Check sheet for the drawn part. Datum: minimum x, y, z corner. Units: mm. A direction names the side the tool comes from. Coordinates: 2 decimals unless noted, no trailing zeros. Order: outer loops, then holes, each group sorted by start corner. A loop starts at its lowest first (then second) coordinate and runs counter-clockwise, first axis right, second up.
1. Set-up check for the marked faces 1, 2 and 3: record each of +Z, -Z, +X, -X, +Y, -Y from which the full face is reachable in a straight line by a thin tool's end or side.
2. Cross-section at A-A (z = 7). Enter the section's corners in (x, y).
3. Cross-section at B-B (x = 4.75). Enter the section's corners in (y, z), then the cut area to 4 significant figures.
4. Gauge pin test, flat ends, axial feed: pin 1 Ø4 at (x, z) = (4.5, 4.5) entering from +Y; pin 2 Ø3 at (x, z) = (4.5, 7) entering from -Y; pin 3 Ø4 at (y, z) = (14.5, 6) entering from +X; pin 4 Ø1.5 at (y, z) = (23.5, 7) entering from -X. Record the tip position at first contact, or that the pin passes through.
5. Draft check along Z on the marked faces 4, 5 and 6. Enter one of: released by +Z, released by -Z, zero draft, split by the parting line, or undercut.
6. Cross-section at C-C (y = 20). Enter the section's corners in (x, z).
7. Thickness scan on line 1 (X direction, y = 2.9, z = 7); line 2 (Y direction, x = 21, z = 7.75); line 3 (Z direction, x = 37, y = 4). Record the ranges inside material, lowest first.
8. Cross-section at D-D (z = 1.75). Enter the section's corners in (x, y).
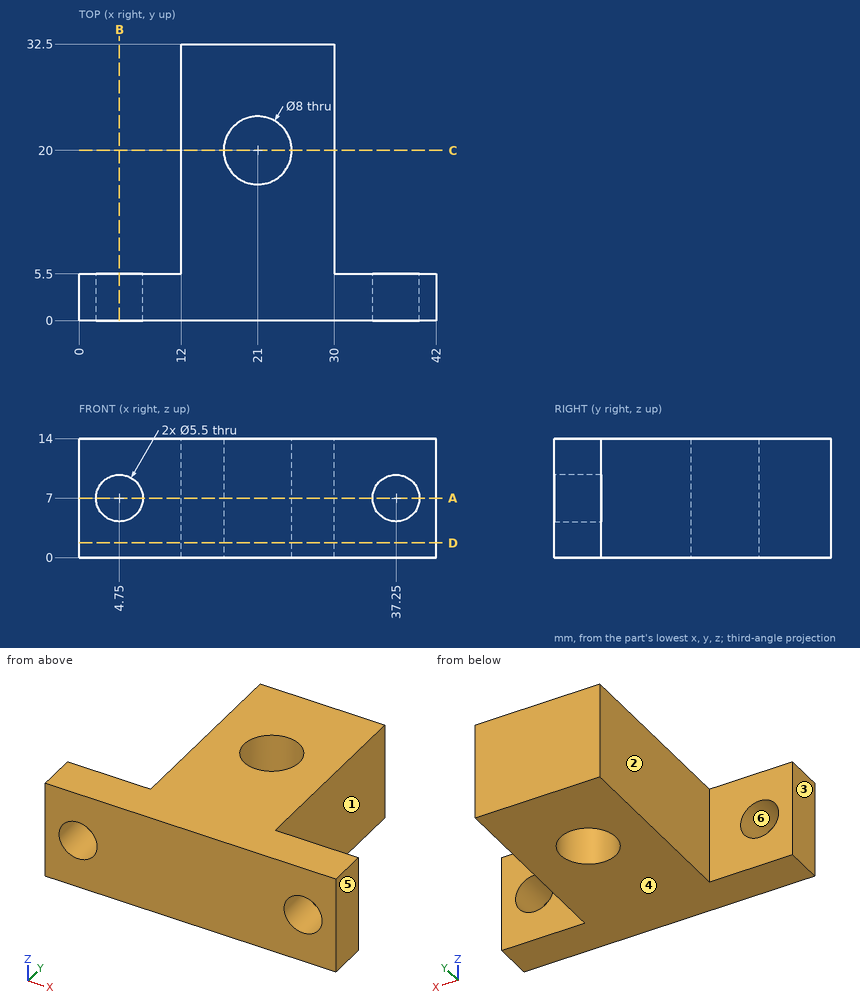
Data:
1. face 1: +Z, -Z, +X, +Y
1. face 2: +Z, -Z, -X, +Y
1. face 3: +Z, -Z, -X, +Y, -Y
2. outline: (0, 0) - (2, 0) - (2, 5.5) - (0, 5.5) - close; (7.5, 0) - (34.5, 0) - (34.5, 5.5) - (30, 5.5) - (30, 32.5) - (12, 32.5) - (12, 5.5) - (7.5, 5.5) - close; (40, 0) - (42, 0) - (42, 5.5) - (40, 5.5) - close; hole circle Ø8 at (21, 20)
3. outline: (0, 0) - (5.5, 0) - (5.5, 4.25) - (0, 4.25) - close; (0, 9.75) - (5.5, 9.75) - (5.5, 14) - (0, 14) - close
3. area: 46.75 mm2
4. pin 1: stops at y = 5.5
4. pin 2: passes through
4. pin 3: stops at x = 30
4. pin 4: stops at x = 12
5. face 4: released by -Z
5. face 5: zero draft
5. face 6: undercut
6. outline: (12, 0) - (17, 0) - (17, 14) - (12, 14) - close; (25, 0) - (30, 0) - (30, 14) - (25, 14) - close
7. line 1: x = 0 to 2, 7.5 to 34.5, 40 to 42
7. line 2: y = 0 to 16, 24 to 32.5
7. line 3: z = 0 to 4.26, 9.74 to 14
8. outline: (0, 0) - (42, 0) - (42, 5.5) - (30, 5.5) - (30, 32.5) - (12, 32.5) - (12, 5.5) - (0, 5.5) - close; hole circle Ø8 at (21, 20)
